from build123d import *

# Parameters (mm, degrees)
SKETCH1_W               = 26
SKETCH1_H               = 26
SKETCH1_W_2             = 20
SKETCH1_H_2             = 20
BOSS_EXTRUDE1_DEPTH     = 30
SKETCH2_W               = 20
SKETCH2_H               = 20
BOSS_EXTRUDE2_DEPTH     = 5
FILLET1_R               = 2
SKETCH6_W               = 3
SKETCH6_H               = 8
BOSS_EXTRUDE4_DEPTH     = 14
FILLET2_R               = 2
FILLET3_R               = 2
SKETCH7_R               = 1.5
CUT_EXTRUDE2_DEPTH      = 10
CUT_EXTRUDE2_DEPTH_BACK = 18
SKETCH9_W               = 23
SKETCH9_H               = 2.5
CUT_EXTRUDE3_DEPTH      = 23
FILLET4_R               = 2


with BuildPart() as part:
    # Sketch1 → Boss-Extrude1 (new body)
    with BuildSketch(Plane(origin=(0, 0, 0), x_dir=(1, 0, 0), z_dir=(0, 1, 0))):
        Rectangle(SKETCH1_W, SKETCH1_H)
        Rectangle(SKETCH1_W_2, SKETCH1_H_2, mode=Mode.SUBTRACT)
    extrude(amount=BOSS_EXTRUDE1_DEPTH)

    # Sketch2 → Boss-Extrude2 (add)
    with BuildSketch(Plane.XZ):
        Rectangle(SKETCH2_W, SKETCH2_H)
    extrude(amount=-BOSS_EXTRUDE2_DEPTH)

    # Fillet1
    fillet1_edges = [part.edges().sort_by_distance(p)[0] for p in [
        (-10, 17.5, -10),
        (-10, 17.5, 10),
        (10, 17.5, 10),
        (10, 17.5, -10),
        (-13, 15, -13),
        (13, 15, -13),
        (13, 15, 13),
        (-13, 15, 13),
    ]]
    fillet(fillet1_edges, radius=FILLET1_R)

    # Sketch6 → Boss-Extrude4 (add)
    with BuildSketch(Plane(origin=(13, 0, 0), x_dir=(0, 0, -1), z_dir=(1, 0, 0))):
        with Locations((-2.5, 15)):
            Rectangle(SKETCH6_W, SKETCH6_H)
        with Locations((2.5, 15)):
            Rectangle(SKETCH6_W, SKETCH6_H)
    extrude(amount=BOSS_EXTRUDE4_DEPTH)

    # Fillet2
    fillet2_edges = [part.edges().sort_by_distance(p)[0] for p in [
        (13, 11, 2.5),
        (13, 19, 2.5),
        (13, 19, -2.5),
        (13, 11, -2.5),
    ]]
    fillet(fillet2_edges, radius=FILLET2_R)

    # Fillet3
    fillet3_edges = [part.edges().sort_by_distance(p)[0] for p in [
        (27, 11, 2.5),
        (27, 19, 2.5),
        (27, 19, -2.5),
        (27, 11, -2.5),
    ]]
    fillet(fillet3_edges, radius=FILLET3_R)

    # Sketch7 → Cut-Extrude2 (cut, two sides)
    with BuildSketch(Plane(origin=(0, 0, -4), x_dir=(-1, 0, 0), z_dir=(0, 0, -1))) as cut_extrude2_sk:
        with Locations((-22.15, 15)):
            Circle(SKETCH7_R)
    extrude(amount=CUT_EXTRUDE2_DEPTH, mode=Mode.SUBTRACT)
    extrude(cut_extrude2_sk.sketch, amount=-CUT_EXTRUDE2_DEPTH_BACK, mode=Mode.SUBTRACT)

    # Sketch9 → Cut-Extrude3 (cut)
    with BuildSketch(Plane.ZY.offset(13)):
        with Locations((0, 26.75)):
            Rectangle(SKETCH9_W, SKETCH9_H)
    extrude(amount=-CUT_EXTRUDE3_DEPTH, mode=Mode.SUBTRACT)

    # Fillet4
    fillet4_edges = [part.edges().sort_by_distance(p)[0] for p in [
        (10, 26.75, 11.5),
        (10, 26.75, -11.5),
    ]]
    fillet(fillet4_edges, radius=FILLET4_R)


solid = part.part
Geometry: final body of the model. Coordinates: model frame, mm. A direction names the side the tool comes from. Give positions to 0.01 mm unless a question says otherwise; leave off trailing zeros. Loops run counter-clockwise (first coordinate to the right, second up) from the corner with the lowest first, then second, coordinate; pieces in that order, holes last. Notation, with made-up numbers: (-1, 22.25) - (13, 22.25) arc R32 cw to (13, 50.25) - close; hole circle Ø1 at (21, -30.5). An arc over 180 degrees is marked (long way). One line per question, with ' | ' between items. Start each with the question number.
(1) Section query B-B on x = 22.15. Return loops of the section in (y, z).
(2) Contact query for flat-ended pins moving along their axis: pin 1 (3.5 mm diameter, centred on x = 18.5, z = 2.5, fed in from +Y); pin 2 (4 mm diameter, centred on x = 16.5, z = -1, fed in from -Y); pin 3 (5 mm diameter, centred on x = 18, z = 5, fed in from -Y). Output: stop coordinate, or through.
(3) Ray query, line 1 (X direction, y = 10, z = 8); line 2 (Z direction, x = 13.5, y = 10.5). Return the intervals inside material, ascending. Write a range as from..to.
(4) Reachability of faces 5 (the flat face through (20, 15, 4)), 6 (the cylindrical face through (-9.4, 29.01, 9.43)), 7 (the cylindrical face through (9.43, 26.77, -10.9)) from +Z, -Z, +X, -X, +Y, -Y: full face, straight path, thin tool, end or side. Return the list, or none.
(5) Section query C-C on z = 1.5. Return loops of the section in (x, y), then the cut area to 3 significant figures.
(6) Pull-direction query (Y, two-part tool) for faces 1 (the flat face through (20, 19, -2)), 2 (the flat face through (0, 29, 10)), 3 (the flat face through (20, 11, 3)), 4 (the cylindrical face through (9.43, 26.77, 10.9)); classes: released by +Y, released by -Y, zero draft, split by the parting line, or undercut.
(7) Section query A-A on y = 15. Count the separate pieces of the cut face and the enclosed holes in it, then the cut area to 3 significant figures.
(8) Section query D-D on x = 0.5. Return loops of the section in (y, z).
The answers:
1) outline: (11, -4) - (13.5, -4) - (13.5, -1) - (11, -1) - close; (11, 1) - (13.5, 1) - (13.5, 4) - (11, 4) - close; (16.5, -4) - (19, -4) - (19, -1) - (16.5, -1) - close; (16.5, 1) - (19, 1) - (19, 4) - (16.5, 4) - close
2) pin 1: y = 19 | pin 2: y = 10.94 | pin 3: y = 11
3) line 1: -13..-10, 10..13 | line 2: -4..-1, 1..4
4) face 5: +Z, +X, +Y, -Y | face 6: +Y | face 7: -X
5) outline: (-13, 0) - (13, 0) - (13, 9) arc R2 cw to (15, 11) - (25, 11) arc R2 ccw to (27, 13) - (27, 17) arc R2 ccw to (25, 19) - (15, 19) arc R2 cw to (13, 21) - (13, 30) - (10, 30) - (10, 5) - (-10, 5) - (-10, 25.5) - (-13, 25.5) - close; (-13, 28) - (-10, 28) - (-10, 30) - (-13, 30) - close; hole circle Ø3 at (22.15, 15) | area: 377 mm2
6) face 1: released by +Y | face 2: zero draft | face 3: released by -Y | face 4: undercut
7) separate pieces: 3 | enclosed holes: 1 | area: 342 mm2
8) outline: (0, -13) - (30, -13) - (30, -10) - (28, -10) - (28, -11.5) - (25.5, -11.5) - (25.5, -10) - (5, -10) - (5, 10) - (25.5, 10) - (25.5, 11.5) - (28, 11.5) - (28, 10) - (30, 10) - (30, 13) - (0, 13) - close
